Could you check a few things on this model? Use its own coordinates, in mm. Coordinates: 2 decimals unless noted, no trailing zeros. Loops run counter-clockwise (first coordinate to the right, second up) from the corner with the lowest first, then second, coordinate; pieces in that order, holes last. Notation, with made-up numbers: (11.25, 40) - (37.25, 40) arc R16 ccw to (37.25, 57) - close; hole circle Ø8 at (49, 54). An arc over 180 degrees is marked (long way). One line per item, written item: value. Start each with the question number.
(1) If I drill on line 1 along X through (y, z) = (-0.25, -124); line 2 along Y through (x, z) = (-4.75, -98) (3 decimals); line 3 along Z through (x, y) = (-6, 1.5), over which ranges is the centre line in solid material (lowest first)? Write a range as from..to.
(2) I'm going to push flat-ended pins straight in: P1, Ø0.6, axis at x = 6, z = -84.5, coming from the +Y side (3 decimals); P2, Ø5, axis at x = -2, y = 0, coming from the +Z side; P3, Ø4, axis at x = 4, y = 0, coming from the +Z side. Where does each tip first touch, or does it pass through?
(3) If we section it at B-B on y = 0: Write out the boundary of the cut face in (x, z).
(4) If we section it at C-C on x = -2.75: Write out the boundary of the cut face in (y, z) (3 decimals), then the cut area to 3 significant figures.
(5) If we section it at A-A on z = -111.5: Write out the boundary of the cut face in (x, y) (3 decimals).
```python
from build123d import *

# Parameters (mm, degrees)
SKETCH1_W           = 12.7
SKETCH1_H           = 6.35
BOSS_EXTRUDE1_DEPTH = 144.78
CUT_EXTRUDE1_DEPTH  = 6.096
SKETCH3_R           = 1.27
BOSS_EXTRUDE2_DEPTH = 0.762
SKETCH5_W           = 12.7
SKETCH5_H           = 6.35
CUT_EXTRUDE2_DEPTH  = 0.762
SKETCH6_W           = 2.54
SKETCH6_H           = 0.254
BOSS_EXTRUDE3_DEPTH = 2.54
SKETCH8_W           = 2.54
SKETCH8_H           = 2.54
CUT_EXTRUDE3_DEPTH  = 2.54


with BuildPart() as part:
    # Sketch1 → Boss-Extrude1 (new body)
    with BuildSketch(Plane.XY):
        Rectangle(SKETCH1_W, SKETCH1_H)
    extrude(amount=-BOSS_EXTRUDE1_DEPTH)

    # Sketch2 → Cut-Extrude1 (cut)
    with BuildSketch(Plane(origin=(0, 3.175, 0), x_dir=(1, 0, 0), z_dir=(0, 1, 0))):
        Polygon((5.588, 0.381), (-5.588, 0.381), (-5.588, 0.762), (-5.588, 144.018), (5.588, 144.018), (5.588, 0.762), align=None)
    extrude(amount=-CUT_EXTRUDE1_DEPTH, mode=Mode.SUBTRACT)

    # Sketch3 → Boss-Extrude2 (add)
    with BuildSketch(Plane(origin=(6.35, 0, 0), x_dir=(0, 0, -1), z_dir=(1, 0, 0))):
        with BuildLine():
            Line((144.78, 3.175), (144.78, 5.979528965))
            Line((144.78, 5.979528965), (144.749123731, 5.979528965))
            ThreePointArc((144.749123731, 5.979528965), (142.844123731, 7.884528965), (140.939123731, 5.979528965))
            Line((140.939123731, 5.979528965), (140.908247462, 5.979528965))
            Line((140.908247462, 5.979528965), (140.908247462, 3.175))
            Line((140.908247462, 3.175), (144.78, 3.175))
        make_face()
        with Locations((142.844123731, 5.979528965)):
            Circle(SKETCH3_R, mode=Mode.SUBTRACT)
    boss_extrude2 = extrude(amount=-BOSS_EXTRUDE2_DEPTH)

    # Mirror1: Boss-Extrude2 across plane
    add(boss_extrude2.mirror(Plane(origin=(0, 0, 0), x_dir=(0, 0, 1), z_dir=(1, 0, 0))))

    # Sketch5 → Cut-Extrude2 (cut)
    with BuildSketch(Plane.XY):
        Rectangle(SKETCH5_W, SKETCH5_H)
    extrude(amount=-CUT_EXTRUDE2_DEPTH, mode=Mode.SUBTRACT)

    # Sketch6 → Boss-Extrude3 (add)
    with BuildSketch(Plane.XY.offset(-0.762)):
        with Locations((0, -3.048)):
            Rectangle(SKETCH6_W, SKETCH6_H)
    extrude(amount=BOSS_EXTRUDE3_DEPTH)

    # Sketch8 → Cut-Extrude3 (cut)
    with BuildSketch(Plane(origin=(0, -2.921, 0), x_dir=(1, 0, 0), z_dir=(0, 1, 0))):
        with Locations((0, 8.382)):
            Rectangle(SKETCH8_W, SKETCH8_H)
    extrude(amount=-CUT_EXTRUDE3_DEPTH, mode=Mode.SUBTRACT)


solid = part.part
```
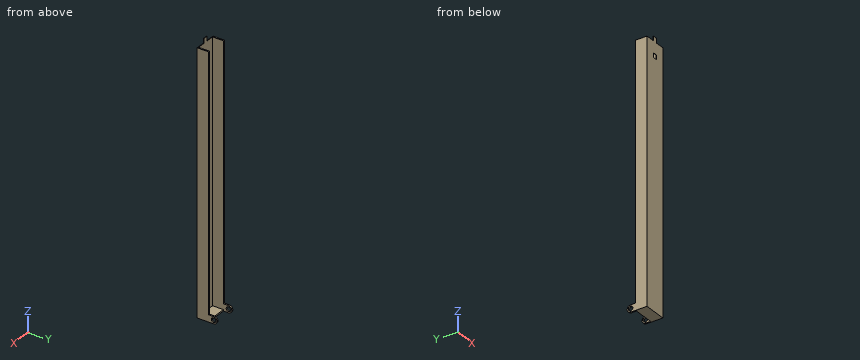
Values:
1. line 1: x = -6.35..-5.59, 5.59..6.35
1. line 2: y = -3.175..-2.921
1. line 3: z = -144.78..-0.76
2. P1: stops at y = 3.175
2. P2: stops at z = -144.02
2. P3: stops at z = -0.76
3. outline: (-6.35, -144.78) - (6.35, -144.78) - (6.35, -0.76) - (5.59, -0.76) - (5.59, -144.02) - (-5.59, -144.02) - (-5.59, -0.76) - (-6.35, -0.76) - close
4. outline: (-3.175, -144.78) - (3.175, -144.78) - (3.175, -144.018) - (-2.921, -144.018) - (-2.921, -0.762) - (-3.175, -0.762) - close
4. area: 41.2 mm2
5. outline: (-6.35, -3.175) - (6.35, -3.175) - (6.35, 3.175) - (5.588, 3.175) - (5.588, -2.921) - (-5.588, -2.921) - (-5.588, 3.175) - (-6.35, 3.175) - close
